Design review of the part built by this model. Coordinates are the model's own, in mm. Face numbers are marked on the shaded views. A direction names the side the tool comes from. Coordinates: 2 decimals unless noted, no trailing zeros. Loops run counter-clockwise (first coordinate to the right, second up) from the corner with the lowest first, then second, coordinate; pieces in that order, holes last. Notation, with made-up numbers: (34, -24) -> (41, -24) arc R24 ccw to (41, -7) -> close; hole circle Ø4 at (75.25, -25). An arc over 180 degrees is marked (long way). One line per item, written item: value. Start each with the question number.
1. Machinability: for the marked faces 1, 2, 3 and 4, which of the approach directions +Z, -Z, +X, -X, +Y, -Y give a long, thin tool a straight path to every point of the face, cutting with its end or side? Answer none if there is none.
2. Add section A-A on y = -6. Write out the cut boundary in (x, z), plus the area to 3 significant figures.
3. Add section C-C on z = 6. Write out the cut boundary in (x, y).
4. Draft analysis for pull direction Z (two halves, no side actions). For the marked faces 5, 6 and 7, state which applies: pulls with the +Z half, pulls with the -Z half, needs draft (parallel to the pull), parting line crosses it, or undercut.
5. Add section B-B on x = 2. Write out the cut boundary in (y, z), plus the area to 3 significant figures.
6. For probe 1 along Z at (x, y) = (12.5, -6.5); probe 2 along Y at (x, z) = (-3, 14.75); probe 3 along Y at (x, z) = (8, 6.75), list the stretches that pass through material, from the lowest coordinate up.
7. Insertion check: pin 1 (1.5 mm diameter, centred on y = -1.5, z = 15.5, fed in from -X); pin 2 (1.1 mm diameter, centred on y = 0.5, z = 8.5, fed in from +X); pin 3 (6 mm diameter, centred on x = 8, z = 6, fed in from +Y); pin 4 (10 mm diameter, centred on x = 10.5, z = 11.5, fed in from -Y). Each pin has a flat end and moves straight along its axis. Give the tip position at first contact, or say it passes through.
8. Add section D-D on x = -7. Write out the cut boundary in (y, z), plus the area to 3 significant figures.
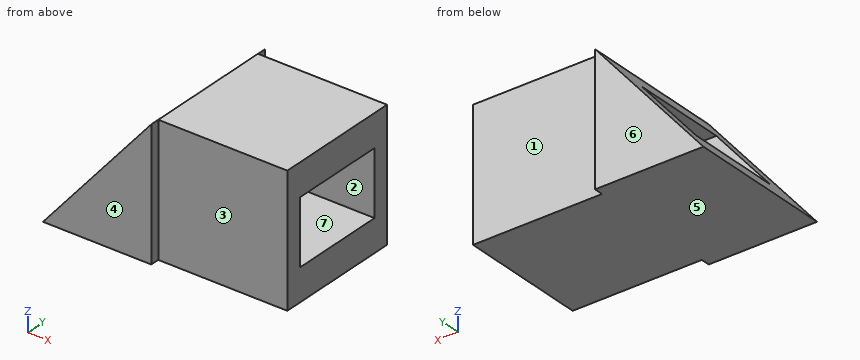
```python
from build123d import *

# Parameters (mm, degrees)
F0_W          = 20
F0_H          = 20
F1_DEPTH      = 20
F2_DEPTH      = 21.4
F2_DEPTH_BACK = 1.4
F3_W          = 15
F3_H          = 10
F4_DEPTH      = 36.782993


with BuildPart() as f1:
    # F0 (on Front) → F1 (new body)
    with BuildSketch(Plane.XZ):
        with Locations((10, 10)):
            Rectangle(F0_W, F0_H)
        Polygon((-16.781993, 0), (0, 0), (0, 20), align=None)
    extrude(amount=F1_DEPTH)

    # F0 (on Front) → F2 (join, two sides)
    with BuildSketch(Plane.XZ) as f2_sk:
        Polygon((-16.781993, 0), (0, 0), (0, 20), align=None)
    extrude(amount=F2_DEPTH)
    extrude(f2_sk.sketch, amount=-F2_DEPTH_BACK)

    # F3 (on face) → F4 (cut, through all)
    with BuildSketch(Plane.YZ.offset(20)):
        with Locations((-10, 10)):
            Rectangle(F3_W, F3_H)
    extrude(amount=-F4_DEPTH, mode=Mode.SUBTRACT)


solid = f1.part
```
Worked answers:
1. face 1: +Z, -Z, +X, +Y
1. face 2: +X, -X
1. face 3: +Z, -Z, +X, -Y
1. face 4: +Z, -Z, +X, -X, -Y
2. outline: (-16.78, 0) -> (20, 0) -> (20, 5) -> (-12.59, 5) -> close; (-4.2, 15) -> (20, 15) -> (20, 20) -> (0, 20) -> close
2. area: 284 mm²
3. outline: (-11.75, -21.4) -> (0, -21.4) -> (0, -20) -> (20, -20) -> (20, -17.5) -> (-11.75, -17.5) -> close; (-11.75, -2.5) -> (20, -2.5) -> (20, 0) -> (0, 0) -> (0, 1.4) -> (-11.75, 1.4) -> close
4. face 5: pulls with the -Z half
4. face 6: needs draft
4. face 7: undercut
5. outline: (-20, 0) -> (0, 0) -> (0, 20) -> (-20, 20) -> close; hole (-17.5, 5) -> (-2.5, 5) -> (-2.5, 15) -> (-17.5, 15) -> close
5. area: 250 mm²
6. probe 1: z = 0 to 5, 15 to 20
6. probe 2: y = -21.4 to -17.5, -2.5 to 1.4
6. probe 3: y = -20 to -17.5, -2.5 to 0
7. pin 1: stops at x = -4.41
7. pin 2: stops at x = 20
7. pin 3: stops at y = 0
7. pin 4: stops at y = -20
8. outline: (-21.4, 0) -> (1.4, 0) -> (1.4, 11.66) -> (-2.5, 11.66) -> (-2.5, 5) -> (-17.5, 5) -> (-17.5, 11.66) -> (-21.4, 11.66) -> close
8. area: 166 mm²
